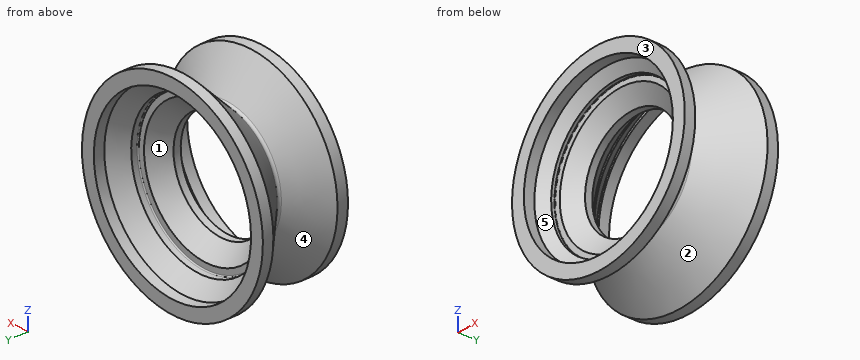
from build123d import *

# Parameters (mm, degrees)
FILLET3_R           = 0.2
FILLET5_R           = 0.1
SKETCH2_R           = 19.042006499
SKETCH2_R_2         = 16.542006499
BOSS_EXTRUDE1_DEPTH = 2
SKETCH3_R           = 18.182746533
SKETCH3_R_2         = 15.682746533
BOSS_EXTRUDE2_DEPTH = 2
MIDDLE_FILLLET_R    = 0.5


with BuildPart() as part:
    # Sketch1 → Revolve1 (revolve)
    with BuildSketch(Plane.XY, mode=Mode.PRIVATE) as revolve1_sk:
        Polygon((-17, 8), (-14.120151906, 5.074731621), (-14.120151906, 3.778145407), (-12.843697628, 3.778145407), (-9.924215024, 0.812617411), (-9.924215024, -0.560166031), (-12.924215024, -2.660788645), (-13.945322255, -2.660788645), (-13.945322255, -3.375775626), (-16.264955058, -5), (-18.182746533, -5), (-11.042006499, 0), (-19.042006499, 8), align=None)
    revolve(revolve1_sk.sketch.rotate(Axis((0, 30.18306827, 0), (0, -1, 0)), 270), axis=Axis((0, 30.18306827, 0), (0, -1, 0)))

    # Fillet3
    fillet3_edges = [part.edges().sort_by_distance(p)[0] for p in [
        (0, 3.778145407, -14.120151906),
    ]]
    fillet(fillet3_edges, radius=FILLET3_R)

    # Fillet5
    fillet5_edges = [part.edges().sort_by_distance(p)[0] for p in [
        (0, -2.660788645, -13.945322255),
    ]]
    fillet(fillet5_edges, radius=FILLET5_R)

    # Sketch2 → Boss-Extrude1 (add)
    with BuildSketch(Plane(origin=(0, 8, 0), x_dir=(1, 0, 0), z_dir=(0, 1, 0))):
        with Locations(Location((0, 0, 0), (0, 0, 270))):
            Circle(SKETCH2_R)
        with Locations(Location((0, 0, 0), (0, 0, 270))):
            Circle(SKETCH2_R_2, mode=Mode.SUBTRACT)
    extrude(amount=BOSS_EXTRUDE1_DEPTH)

    # Sketch3 → Boss-Extrude2 (add)
    with BuildSketch(Plane.XZ.offset(5)):
        with Locations(Location((0, 0, 0), (0, 0, 270))):
            Circle(SKETCH3_R)
        with Locations(Location((0, 0, 0), (0, 0, 270))):
            Circle(SKETCH3_R_2, mode=Mode.SUBTRACT)
    extrude(amount=BOSS_EXTRUDE2_DEPTH)

    # middle_filllet
    middle_filllet_edges = [part.edges().sort_by_distance(p)[0] for p in [
        (0, 0, -11.042006499),
    ]]
    fillet(middle_filllet_edges, radius=MIDDLE_FILLLET_R)


solid = part.part
The listing builds one solid part. Answer for the finished solid, in the listing's coordinates (mm). Face numbers are marked on the shaded views. A direction names the side the tool comes from. Give positions to 0.01 mm unless a question says otherwise; leave off trailing zeros. Write each loop counter-clockwise with the first axis right and the second up, starting at its lowest first coordinate (ties: lowest second). Pieces come first, ordered by that corner, then holes. Notation, with made-up numbers: (-25.75, 86.25) - (-16.75, 86.25) arc R20 cw to (-16.75, 109.25) - close; hole circle Ø10 at (-16.75, 23.25). An arc over 180 degrees is marked (long way). Use a Markdown table: item, result.
1. Find the intervals of material crossed by probe 1 along Y at (x, z) = (-13, -2.5); probe 2 along Y at (x, z) = (9, 13); probe 3 along X at (y, z) = (9, -4), in increasing order. Write a range as from..to.
Values follow:
| item | result |
|---|---|
| probe 1 | y = -2.66..-1.54, 2.2..3.78 |
| probe 2 | y = -7..-5, -4.68..-3.34, 4.77..6.79 |
| probe 3 | x = -18.62..-16.05, 16.05..18.62 |
2. For a pull along X with two mould halves and no side action, classify the marked faces 3, 4 and 5 as released by +X, released by -X, zero draft, split by the parting line, or undercut.
Values follow:
| item | result |
|---|---|
| face 3 | zero draft |
| face 4 | split by the parting line |
| face 5 | undercut |
3. Section A-A on y = 2.5 is taken. Write down the section's boundary in (x, z).
Values follow:
| item | result |
|---|---|
| outline | circle Ø27.08 at (0, 0); hole circle Ø23.17 at (0, 0) |
4. A tool of negligible diameter and unlimited length cuts with its end or side. For the marked faces 1 and 2, from which of +Z, -Z, +X, -X, +Y, -Y can it reach the whole face along a straight path? Write none if from no direction.
Values follow:
| item | result |
|---|---|
| face 1 | +Y |
| face 2 | none |
5. Each of these flat-tipped pins is pushed along its axis until it touches: P1, Ø1, axis at x = -4.5, y = -3.5, coming from the +Z side; P2, Ø1.5, axis at x = 2, y = 0, coming from the +Z side; P3, Ø10, axis at x = -4, y = 2.5, coming from the -Z side. Where does it stop, or does it pass through?
Values follow:
| item | result |
|---|---|
| P1 | stops at z = 16.15 |
| P2 | stops at z = 11.95 |
| P3 | stops at z = -18.2 |
6. Section B-B on y = -2 is taken. Write down the section's boundary in (x, z), plus the area to 3 significant figures.
Values follow:
| item | result |
|---|---|
| outline | circle Ø27.8 at (0, 0); hole circle Ø23.96 at (0, 0) |
| area | 156 mm² |
